from build123d import *

# Parameters (mm, degrees)
EXTRUDE_THIN1_DEPTH = 25.4
SKETCH2_R           = 3.81
CUT_EXTRUDE1_DEPTH  = 8.128


with BuildPart() as part:
    # Sketch1 → Extrude-Thin1 (new, symmetric)
    with BuildSketch(Plane.XY):
        with BuildLine():
            Line((29.4005, 0), (16.7005, 0))
            ThreePointArc((16.7005, 0), (0, -16.7005), (-16.7005, 0))
            Line((-16.7005, 0), (-29.4005, 0))
            Line((-29.4005, 0), (-29.4005, -2.54))
            Line((-29.4005, -2.54), (-19.07210634, -2.54))
            ThreePointArc((-19.07210634, -2.54), (0, -19.2405), (19.07210634, -2.54))
            Line((19.07210634, -2.54), (29.4005, -2.54))
            Line((29.4005, -2.54), (29.4005, 0))
        make_face()
    extrude(amount=EXTRUDE_THIN1_DEPTH, both=True)

    # Sketch2 → Cut-Extrude1 (cut)
    with BuildSketch(Plane.XZ.offset(2.54)):
        with Locations(Location((24.23630317, -12.7, 0), (0, 0, 270))):
            Circle(SKETCH2_R)
        with Locations(Location((24.23630317, 12.7, 0), (0, 0, 270))):
            Circle(SKETCH2_R)
        with Locations(Location((-24.27769683, 12.7, 0), (0, 0, 270))):
            Circle(SKETCH2_R)
        with Locations(Location((-24.27769683, -12.7, 0), (0, 0, 270))):
            Circle(SKETCH2_R)
    extrude(amount=-CUT_EXTRUDE1_DEPTH, mode=Mode.SUBTRACT)


solid = part.part
Design review of the part built by this model. Coordinates are the model's own, in mm. A direction names the side the tool comes from. Round coordinates to 2 decimals unless told otherwise and drop trailing zeros. Write each loop counter-clockwise with the first axis right and the second up, starting at its lowest first coordinate (ties: lowest second). Pieces come first, ordered by that corner, then holes. Notation, with made-up numbers: M 43.25,-35.75 L 51.25,-35.75 A20 cw 51.25,-8.75 Z; hole C 78,-36 d6. An arc over 180 degrees is marked long. One line per item, written item: value. Start each with the question number.
1. Draft analysis for pull direction X (two halves, no side actions). For faces 4 (the face through (-0.387, -19.237, 0.356)), 5 (the face through (-24.11, -1.288, 16.506)), 6 (the face through (23, 0, 0)), 7 (the face through (24.404, -1.288, 16.506)), state which applies: pulls with the +X half, pulls with the -X half, needs draft (parallel to the pull), parting line crosses it, or undercut.
2. Take a section at C-C on y = -12.25. State the section outline as (x, z) points, then the cut area to 3 significant figures.
3. Take a section at D-D on z = 20. State the section outline as (x, y) points, then the cut area to 3 significant figures.
4. Take a section at B-B on x = 22.5. State the section outline as (y, z) points.
5. Take a section at A-A on z = -12.7. State the section outline as (x, y) points, then the cut area to 3 significant figures.
6. Clearance check with flat-ended pins moving along their axes: P1, Ø11.5, axis at x = -26.5, z = 6.5, coming from the -Y side; P2, Ø8, axis at x = 12.5, z = -1.5, coming from the -Y side; P3, Ø1, axis at y = -14.5, z = 3, coming from the +X side. State where each tip first meets the part, or that it passes through.
7. To check wall thickness, follow probe 1 along X at (y, z) = (-1.55, -12.7); probe 2 along X at (y, z) = (-1, -12.7); probe 3 along Y at (x, z) = (-24.5, 3.5). State the ranges of each line that lie inside material, in increasing order. Write a range as from..to.
8. For faces 1 (the face through (-24, -2.54, 0)), 2 (the face through (24, -2.54, 0)), 3 (the face through (-29.4, -1, 0)), list the 3-axis set-ups (+Z, -Z, +X, -X, +Y, -Y) from which the entire face can be reached by the end or side of a thin tool; tool diameter is ignored.
Computed:
1. face 4: parting line crosses it
1. face 5: undercut
1. face 6: needs draft
1. face 7: undercut
2. outline: M -14.84,-25.4 L -11.35,-25.4 L -11.35,25.4 L -14.84,25.4 Z; M 11.35,-25.4 L 14.84,-25.4 L 14.84,25.4 L 11.35,25.4 Z
2. area: 354 mm²
3. outline: M -29.4,-2.54 L -19.07,-2.54 A19.24 ccw 19.07,-2.54 L 29.4,-2.54 L 29.4,0 L 16.7,0 A16.7 cw -16.7,0 L -29.4,0 Z
3. area: 195 mm²
4. outline: M -2.54,-25.4 L 0,-25.4 L 0,-16.09 L -2.54,-16.09 Z; M -2.54,-9.31 L 0,-9.31 L 0,9.31 L -2.54,9.31 Z; M -2.54,16.09 L 0,16.09 L 0,25.4 L -2.54,25.4 Z
5. outline: M -29.4,-2.54 L -28.09,-2.54 L -28.09,0 L -29.4,0 Z; M -20.47,-2.54 L -19.07,-2.54 A19.24 ccw 19.07,-2.54 L 20.43,-2.54 L 20.43,0 L 16.7,0 A16.7 cw -16.7,0 L -20.47,0 Z; M 28.05,-2.54 L 29.4,-2.54 L 29.4,0 L 28.05,0 Z
5. area: 157 mm²
6. P1: stops at y = -2.54
6. P2: stops at y = -17.26
6. P3: stops at x = 13.2
7. probe 1: x = -29.4..-28.09, -20.47..-16.63, 16.63..20.43, 28.05..29.4
7. probe 2: x = -29.4..-28.09, -20.47..-16.67, 16.67..20.43, 28.05..29.4
7. probe 3: y = -2.54..0
8. face 1: +Z, -Z, -X, -Y
8. face 2: +Z, -Z, +X, -Y
8. face 3: +Z, -Z, -X, +Y, -Y
